CAD build for the part. Positions are in the model's coordinates, mm. A direction names the side the tool comes from. Coordinates: 2 decimals unless noted, no trailing zeros. Write each loop counter-clockwise with the first axis right and the second up, starting at its lowest first coordinate (ties: lowest second). Pieces come first, ordered by that corner, then holes. Notation, with made-up numbers: M 78,-36.5 L 117,-36.5 A15 cw 117,-31.5 Z; hole C 4.5,54.25 d2. An arc over 180 degrees is marked long. Put each result on its own line as item: value. Start each with the question number.
```python
from build123d import *

# Parameters (mm, degrees)
EXTRUDE_THIN1_DEPTH = 430
SKETCH2_R           = 2.1
CUT_EXTRUDE1_DEPTH  = 10


with BuildPart() as part:
    # Sketch1 → Extrude-Thin1 (new body)
    with BuildSketch(Plane(origin=(0, 0, 0), x_dir=(1, 0, 0), z_dir=(0, 1, 0))):
        Polygon((-10.945454545, 0), (-10.945454545, 7.7), (6.054545455, 7.7), (6.054545455, 0), (5.054545455, 0), (5.054545455, 6.7), (-9.945454545, 6.7), (-9.945454545, 0), align=None)
    extrude(amount=EXTRUDE_THIN1_DEPTH)

    # Sketch2 → Cut-Extrude1 (cut)
    with BuildSketch(Plane.XY.offset(-6.7)):
        with Locations((-2.445454545, 390)):
            Circle(SKETCH2_R)
        with Locations(Location((-2.445454545, 40, 0), (0, 0, 180))):
            Circle(SKETCH2_R)
    extrude(amount=-CUT_EXTRUDE1_DEPTH, mode=Mode.SUBTRACT)


solid = part.part
```
(1) Which spindle directions (+Z, -Z, +X, -X, +Y, -Y) get a long thin tool onto all of the face, cutting with end or side? Do faces 1 (the face through (-2, 212, -6.7)), 2 (the face through (-2, 0, -7)). Say none if no direction does.
(2) Drill centre lines: line 1 (X direction, y = 347, z = -4.25); line 2 (X direction, y = 390, z = -7.5); line 3 (Z direction, x = 4.25, y = 35.5). Where is each one in solid material? Low to high. Write a range as [from, to].
(3) Slice it at A-A, the plane z = -3. Write the cut outline in (x, y), then the cut area to 3 significant figures.
(4) Two-plate mould, pull along X, no slides. Class faces 3 (the face through (6.055, 212, -4)), 4 (the face through (5.055, 212, -3)), 5 (the face through (-9.945, 212, -3)), 6 (the face through (-10.945, 212, -4)): +X half, -X half, draft (parallel to the pull), parting line (faces both ways), or undercut.
(5) Slice it at B-B, the plane y = 245.5. Write the cut outline in (x, z), then the cut area to 3 significant figures.
(6) Drop a flat-ended pin along its axis: pin 1 (2 mm diameter, centred on x = -1.5, y = 247, fed in from +Z). Give the stop position or say it passes through.
Result set:
1. face 1: +Z, +Y, -Y
1. face 2: +Z, -Z, +X, -X, -Y
2. line 1: x = [-10.95, -9.95], [5.05, 6.05]
2. line 2: x = [-10.95, -4.55], [-0.35, 6.05]
2. line 3: z = [-7.7, -6.7]
3. outline: M -10.95,0 L -9.95,0 L -9.95,430 L -10.95,430 Z; M 5.05,0 L 6.05,0 L 6.05,430 L 5.05,430 Z
3. area: 860 mm^2
4. face 3: +X half
4. face 4: undercut
4. face 5: undercut
4. face 6: -X half
5. outline: M -10.95,-7.7 L 6.05,-7.7 L 6.05,0 L 5.05,0 L 5.05,-6.7 L -9.95,-6.7 L -9.95,0 L -10.95,0 Z
5. area: 30.4 mm^2
6. pin 1: stops at z = -6.7
